from build123d import *

# Parameters (mm, degrees)
BOSS_EXTRUDE1_DEPTH = 25
SKETCH2_R           = 2
BOSS_EXTRUDE2_DEPTH = 5
SKETCH3_R           = 1.75
CUT_EXTRUDE1_DEPTH  = 5
SKETCH4_R           = 2.6
CUT_EXTRUDE2_DEPTH  = 2.1
BOSS_EXTRUDE4_DEPTH = 1.5
SKETCH6_R           = 8.5
SKETCH6_W           = 11
SKETCH6_H           = 3
CUT_EXTRUDE3_DEPTH  = 62.991888409
SKETCH7_R           = 8.5
SKETCH7_W           = 11
SKETCH7_H           = 4
CUT_EXTRUDE4_DEPTH  = 62.991888409
CUT_EXTRUDE6_DEPTH  = 2
CUT_EXTRUDE7_DEPTH  = 3.5


with BuildPart() as part:
    # Sketch1 → Boss-Extrude1 (new body)
    with BuildSketch(Plane(origin=(0, 0, 0), x_dir=(1, 0, 0), z_dir=(0, 1, 0))):
        Polygon((0, 0), (-48.296291314, -12.940952255), (-47.261015134, -16.80465556), (0, -4.141104722), (47.261015134, -16.80465556), (48.296291314, -12.940952255), align=None)
    extrude(amount=BOSS_EXTRUDE1_DEPTH)

    # Sketch2 → Boss-Extrude2 (add)
    with BuildSketch(Plane(origin=(0, 25, 0), x_dir=(1, 0, 0), z_dir=(0, 1, 0))):
        Polygon((18.842355233, -29.75672149), (-18.842355233, -29.75672149), (-31.057618335, -29.75672149), (-35.381056589, -13.621430262), (0, -4.141104722), (35.381056589, -13.621430262), (31.057618335, -29.75672149), align=None)
        with Locations(Location((-12, -21.75672149, 0), (0, 0, 270))):
            Circle(SKETCH2_R, mode=Mode.SUBTRACT)
        with Locations(Location((12, -21.75672149, 0), (0, 0, 270))):
            Circle(SKETCH2_R, mode=Mode.SUBTRACT)
    extrude(amount=-BOSS_EXTRUDE2_DEPTH)

    # Sketch3 → Cut-Extrude1 (cut)
    with BuildSketch(Plane(origin=(0, 25, 0), x_dir=(1, 0, 0), z_dir=(0, 1, 0))):
        Polygon((24.5917878, -13.318644854), (23.220046861, -18.438051734), (25.345083679, -19.007453633), (26.716824618, -13.888046753), align=None)
        with Locations(Location((21.104732435, -15.127773063, 0), (0, 0, 270))):
            Circle(SKETCH3_R)
        Polygon((18.989418008, -11.817494393), (17.617677069, -16.936901272), (15.492640251, -16.367499373), (16.86438119, -11.248092493), align=None)
        Polygon((-15.492640251, -16.367499373), (-17.617677069, -16.936901272), (-18.989418008, -11.817494393), (-16.86438119, -11.248092493), align=None)
        with Locations(Location((-21.104732435, -15.127773063, 0), (0, 0, 270))):
            Circle(SKETCH3_R)
        Polygon((-25.345083679, -19.007453633), (-26.716824618, -13.888046753), (-24.5917878, -13.318644854), (-23.220046861, -18.438051734), align=None)
    extrude(amount=-CUT_EXTRUDE1_DEPTH, mode=Mode.SUBTRACT)

    # Sketch4 → Cut-Extrude2 (cut)
    with BuildSketch(Plane(origin=(0, 25, 0), x_dir=(1, 0, 0), z_dir=(0, 1, 0))):
        with Locations(Location((-21.104732435, -15.127773063, 0), (0, 0, 270))):
            Circle(SKETCH4_R)
        with Locations(Location((21.104732435, -15.127773063, 0), (0, 0, 270))):
            Circle(SKETCH4_R)
    extrude(amount=-CUT_EXTRUDE2_DEPTH, mode=Mode.SUBTRACT)

    # Sketch5 → Boss-Extrude4 (add)
    with BuildSketch(Plane(origin=(0, 25, 0), x_dir=(1, 0, 0), z_dir=(0, 1, 0))):
        Polygon((-26.716824618, -13.888046753), (-25.345083679, -19.007453633), (-23.220046861, -18.438051734), (-24.5917878, -13.318644854), align=None)
        Polygon((-17.617677069, -16.936901272), (-15.492640251, -16.367499373), (-16.86438119, -11.248092493), (-18.989418008, -11.817494393), align=None)
        Polygon((18.989418008, -11.817494393), (17.617677069, -16.936901272), (15.492640251, -16.367499373), (16.86438119, -11.248092493), align=None)
        Polygon((24.5917878, -13.318644854), (26.716824618, -13.888046753), (25.345083679, -19.007453633), (23.220046861, -18.438051734), align=None)
    extrude(amount=-BOSS_EXTRUDE4_DEPTH)

    # Sketch6 → Cut-Extrude3 (cut, through all)
    with BuildSketch(Plane(origin=(0, 0, 0), x_dir=(-0.9659258262890691, 0, 0.2588190451025181), z_dir=(-0.2588190451025181, 0, -0.9659258262890691))):
        with Locations((37.2, 10)):
            Circle(SKETCH6_R)
        with Locations((11.2, 10)):
            Circle(SKETCH6_R)
        with Locations((24.5, 17.7)):
            Rectangle(SKETCH6_W, SKETCH6_H)
    extrude(amount=-CUT_EXTRUDE3_DEPTH, mode=Mode.SUBTRACT)

    # Sketch7 → Cut-Extrude4 (cut, through all)
    with BuildSketch(Plane(origin=(0, 0, 0), x_dir=(-0.9659258262890691, 0, -0.2588190451025176), z_dir=(0.25881904510251763, 0, -0.9659258262890692))):
        with Locations((-10.82, 10)):
            Circle(SKETCH7_R)
        with Locations((-37.2, 10)):
            Circle(SKETCH7_R)
        with Locations((-24, 17.2)):
            Rectangle(SKETCH7_W, SKETCH7_H)
    extrude(amount=-CUT_EXTRUDE4_DEPTH, mode=Mode.SUBTRACT)

    # Sketch8 → Cut-Extrude6 (cut)
    with BuildSketch(Plane(origin=(0, 0, 0), x_dir=(-1, 0, 0), z_dir=(0, -1, 0))):
        Polygon((-29.167865413, -11.956610704), (-15.363800523, -8.257822665), (-16.010848136, -5.843008099), (-29.814913026, -9.541796138), align=None)
        Polygon((15.363800523, -8.257822665), (29.852687918, -12.140108341), (30.499735531, -9.725293775), (16.010848136, -5.843008099), align=None)
    extrude(amount=-CUT_EXTRUDE6_DEPTH, mode=Mode.SUBTRACT)

    # Sketch9 → Cut-Extrude7 (cut)
    with BuildSketch(Plane(origin=(0, 20, 0), x_dir=(-1, 0, 0), z_dir=(0, -1, 0))):
        Polygon((-25.086264634, -19.973379459), (-22.961227816, -19.40397756), (-23.220046861, -18.438051734), (-25.345083679, -19.007453633), align=None)
        Polygon((-15.492640251, -16.367499373), (-15.233821206, -17.333425199), (-17.358858024, -17.902827098), (-17.617677069, -16.936901272), align=None)
        Polygon((15.233821206, -17.333425199), (17.358858024, -17.902827098), (17.617677069, -16.936901272), (15.492640251, -16.367499373), align=None)
        Polygon((25.345083679, -19.007453633), (25.086264634, -19.973379459), (22.961227816, -19.40397756), (23.220046861, -18.438051734), align=None)
    extrude(amount=-CUT_EXTRUDE7_DEPTH, mode=Mode.SUBTRACT)


solid = part.part
Geometry check sheet. Reference: the model listing, model coordinates, mm. A direction names the side the tool comes from. Give positions to 0.01 mm unless a question says otherwise; leave off trailing zeros. Order: outer loops, then holes, each group sorted by start corner. A loop starts at its lowest first (then second) coordinate and runs counter-clockwise, first axis right, second up. Notation, with made-up numbers: M 88,32 L 125,32 A15 cw 125,42 Z; hole C 36.25,-6.75 d5. An arc over 180 degrees is marked long. Use a Markdown table: item, result.
Item 1: Material ranges on line 1 along Y through (x, z) = (19, 7.75); line 2 along Y through (x, z) = (28, 15.5); line 3 along X through (y, z) = (24, 22.5), recorded low to high.
Answers follow:
| item | result |
|---|---|
| line 1 | y = 2 to 15.2, 19.2 to 25 |
| line 2 | y = 20 to 25 |
| line 3 | x = -33 to -13.86, -10.14 to 10.14, 13.86 to 33 |
Item 2: Section check C-C (y = 8.75). Record the cut outline in (x, z).
Answers follow:
| item | result |
|---|---|
| outline | M -48.3,12.94 L -44.05,11.8 L -43.02,15.67 L -47.26,16.8 Z; M -27.81,7.45 L -18.94,5.07 L -17.9,8.94 L -26.78,11.32 Z; M -2.7,0.72 L 0,0 L 2.33,0.62 L 1.29,4.49 L 0,4.14 L -1.66,4.59 Z; M 17.54,8.84 L 18.57,4.98 L 27.81,7.45 L 26.78,11.32 Z; M 43.02,15.67 L 44.05,11.8 L 48.3,12.94 L 47.26,16.8 Z |
Item 3: Depth check by flat-ended pin: P1, Ø1.5, axis at y = 20, z = 16, coming from the +X side; P2, Ø4, axis at x = -17, z = 15, coming from the -Y side; P3, Ø10, axis at x = 12.5, y = 21, coming from the -Z side; P4, Ø3.5, axis at x = 24, z = 9.5, coming from the -Y side. Enter the tip coordinate at first touch or a pass-through.
Answers follow:
| item | result |
|---|---|
| P1 | stops at x = 47.68 |
| P2 | stops at y = 20 |
| P3 | stops at z = 2.01 |
| P4 | stops at y = 0 |
Item 4: Draft check along X on faces 6 (the flat face through (-17, 23.5, 15)), 7 (the flat face through (24.039, 21.726, 19.693)), 8 (the flat face through (-47.8, 12.3, 14.8)), 9 (the flat face through (0, 23, 29.757)). Enter one of: +X half, -X half, draft (parallel to the pull), parting line (faces both ways), or undercut.
Answers follow:
| item | result |
|---|---|
| face 6 | undercut |
| face 7 | undercut |
| face 8 | -X half |
| face 9 | draft |
Item 5: Section check A-A (y = 13.25). Record the cut outline in (x, z).
Answers follow:
| item | result |
|---|---|
| outline | M -48.3,12.94 L -43.52,11.66 L -42.48,15.52 L -47.26,16.8 Z; M -28.35,7.6 L -18.4,4.93 L -17.37,8.8 L -27.31,11.46 Z; M -3.23,0.87 L 0,0 L 2.86,0.77 L 1.83,4.63 L 0,4.14 L -2.2,4.73 Z; M 17,8.7 L 18.04,4.83 L 28.35,7.6 L 27.31,11.46 Z; M 42.48,15.52 L 43.52,11.66 L 48.3,12.94 L 47.26,16.8 Z |
Item 6: Section check D-D (x = -12). State how many separate pieces and enclosed holes the cut face has, and give its area (3 significant figures).
Answers follow:
| item | result |
|---|---|
| separate pieces | 3 |
| enclosed holes | 0 |
| area | 127 mm2 |
Item 7: Tool access check on faces 1 (the cylindrical face through (-8.53, 1.7, 4.33)), 2 (the flat face through (-23, 22.9, 16)), 3 (the flat face through (23.3, 9.547, 10.384)), 4 (the flat face through (-30.17, 0.99, 10.95)), 5 (the flat face through (-33.19, 22.54, 21.8)). Record the directions out of +Z, -Z, +X, -X, +Y, -Y that give a thin tool (end or side, any length) a straight path to the whole face; none if there is none.
Answers follow:
| item | result |
|---|---|
| face 1 | none |
| face 2 | +Y |
| face 3 | +Z, -Y |
| face 4 | -Y |
| face 5 | +Z, +Y, -Y |
Item 8: Section check B-B (z = 21.75). Record the cut outline in (x, y), and give its area (3 significant figures).
Answers follow:
| item | result |
|---|---|
| outline | M -33.2,20 L -14,20 L -14,25 L -33.2,25 Z; M -10,20 L 10,20 L 10,25 L -10,25 Z; M 14,20 L 33.2,20 L 33.2,25 L 14,25 Z |
| area | 292 mm2 |
